Design review of the part built by this model. Coordinates are the model's own, in mm. Face numbers are marked on the shaded views. Round coordinates to 2 decimals unless told otherwise and drop trailing zeros. Loops run counter-clockwise (first coordinate to the right, second up) from the corner with the lowest first, then second, coordinate; pieces in that order, holes last. Notation, with made-up numbers: M 33,-2 L 78,-2 A10 ccw 78,17 Z; hole C -33,-27.5 d9. An arc over 180 degrees is marked long. One line per item, written item: value. Start each with the question number.
Item 1: For line 1 along X through (y, z) = (20, -4.5); line 2 along Y through (x, z) = (19.05, -51.5) (3 decimals); line 3 along X through (y, z) = (33.5, -23), list the stretches that pass through material, from the lowest coordinate up.
Item 2: Mouldability with a two-part tool opening along X and no side actions: class the marked faces 1, 2 and 3 as released by +X, released by -X, zero draft, split by the parting line, or undercut.
Item 3: Clearance check with flat-ended pins moving along their axes: pin 1 (5.5 mm diameter, centred on x = 33.32, y = 3.94, fed in from -Z); pin 2 (1 mm diameter, centred on y = 15.5, z = -64, fed in from +X); pin 3 (15 mm diameter, centred on x = 17, y = 26, fed in from +Z). State where each tip first meets the part, or that it passes through.
Item 4: We need section A-A (x = 23.5). Write out the cut boundary in (y, z) (3 decimals).
Item 5: We need section C-C (z = -46.5). Write out the cut boundary in (x, y) (3 decimals).
Item 6: We need section B-B (y = 9). Write out the cut boundary in (x, z).
from build123d import *

# Parameters (mm, degrees)
F0_W     = 38.1
F0_H     = 39.624
F1_DEPTH = 4.826
F2_R     = 15.875
F3_DEPTH = 89.916
F4_R     = 15.113
F5_DEPTH = 88.392
F6_R     = 2.0828
F7_DEPTH = 89.917


with BuildPart() as f1:
    # F0 (on Top) → F1 (new body)
    with BuildSketch(Plane.XY):
        with Locations((19.05, 19.812)):
            Rectangle(F0_W, F0_H)
    extrude(amount=-F1_DEPTH)

    # F2 (on face) → F3 (join)
    with BuildSketch(Plane.XY):
        with Locations((19.05, 19.812)):
            Circle(F2_R)
    extrude(amount=-F3_DEPTH)

    # F4 (on face) → F5 (cut)
    with BuildSketch(Plane.XY):
        with Locations((19.05, 19.812)):
            Circle(F4_R)
    extrude(amount=-F5_DEPTH, mode=Mode.SUBTRACT)

    # F6 (on Top) → F7 (cut, through all)
    with BuildSketch(Plane.XY):
        with Locations((33.3248, 35.687)):
            Circle(F6_R)
        with Locations((33.3248, 3.937)):
            Circle(F6_R)
        with Locations((4.7498, 35.687)):
            Circle(F6_R)
        with Locations((4.7498, 3.937)):
            Circle(F6_R)
    extrude(amount=-F7_DEPTH, mode=Mode.SUBTRACT)


solid = f1.part
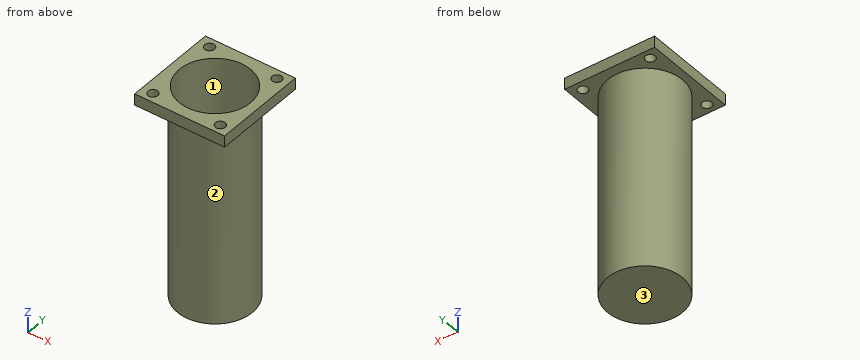
A:
1. line 1: 0 to 3.94, 34.16 to 38.1
1. line 2: 3.937 to 4.699, 34.925 to 35.687
1. line 3: 11.01 to 12.64, 25.46 to 27.09
2. face 1: undercut
2. face 2: split by the parting line
2. face 3: zero draft
3. pin 1: z = -4.83
3. pin 2: x = 34.46
3. pin 3: z = -88.39
4. outline: M 0,-4.826 L 4.573,-4.826 L 4.573,-89.916 L 35.051,-89.916 L 35.051,-4.826 L 39.624,-4.826 L 39.624,0 L 34.255,0 L 34.255,-88.392 L 5.369,-88.392 L 5.369,0 L 0,0 Z
5. outline: C 19.05,19.812 d31.75; hole C 19.05,19.812 d30.226
6. outline: M 0,-4.83 L 7.43,-4.83 L 7.43,-89.92 L 30.67,-89.92 L 30.67,-4.83 L 38.1,-4.83 L 38.1,0 L 29.61,0 L 29.61,-88.39 L 8.49,-88.39 L 8.49,0 L 0,0 Z
